```python
from build123d import *

# Parameters (mm, degrees)
SKIZZE1_W                            = 100
SKIZZE1_H                            = 50
SKIZZE1_W_2                          = 20
SKIZZE1_H_2                          = 3
AUFSATZ_LINEAR_AUSTRAGEN1_DEPTH      = 3
SKIZZE2_W                            = 90
SKIZZE2_H                            = 25
AUFSATZ_LINEAR_AUSTRAGEN2_DEPTH      = 5
SCHNITT_LINEAR_AUSTRAGEN1_DEPTH      = 4
SKIZZE4_W                            = 6
SKIZZE4_H                            = 16
SCHNITT_LINEAR_AUSTRAGEN2_DEPTH      = 5
SCHNITT_LINEAR_AUSTRAGEN2_DEPTH_BACK = 5
SKIZZE5_W                            = 25
SKIZZE5_H                            = 12.5
SCHNITT_LINEAR_AUSTRAGEN3_DEPTH      = 5.6
SKIZZE6_W                            = 4
SKIZZE6_H                            = 12.5
SCHNITT_LINEAR_AUSTRAGEN4_DEPTH      = 6.6
SCHNITT_LINEAR_AUSTRAGEN4_DEPTH_BACK = 3.4
SKIZZE8_W                            = 13
SKIZZE8_H                            = 20.5
SCHNITT_LINEAR_AUSTRAGEN5_DEPTH      = 5
SKIZZE9_W                            = 10
SKIZZE9_H                            = 20.5
SCHNITT_LINEAR_AUSTRAGEN6_DEPTH      = 8
AUFSATZ_LINEAR_AUSTRAGEN3_DEPTH      = 1
AUFSATZ_LINEAR_AUSTRAGEN4_DEPTH      = 17
SKIZZE14_W                           = 3
SKIZZE14_H                           = 42
AUFSATZ_LINEAR_AUSTRAGEN5_DEPTH      = 3
SKIZZE15_W                           = 3
SKIZZE15_H                           = 16
SCHNITT_LINEAR_AUSTRAGEN7_DEPTH      = 3
SKIZZE16_W                           = 2
SKIZZE16_H                           = 2
AUFSATZ_LINEAR_AUSTRAGEN6_DEPTH      = 17
SKIZZE17_W                           = 2
SKIZZE17_H                           = 40
SCHNITT_LINEAR_AUSTRAGEN8_DEPTH      = 20
SKIZZE18_W                           = 35
SKIZZE18_H                           = 2
SCHNITT_LINEAR_AUSTRAGEN9_DEPTH      = 17
SKIZZE19_W                           = 2
SKIZZE19_H                           = 6
SKIZZE19_W_2                         = 4
SKIZZE19_H_2                         = 4
AUFSATZ_LINEAR_AUSTRAGEN7_DEPTH      = 17
SKIZZE20_W                           = 1
SKIZZE20_H                           = 42
AUFSATZ_LINEAR_AUSTRAGEN8_DEPTH      = 3
SKIZZE21_W                           = 2
SKIZZE21_H                           = 3
AUFSATZ_LINEAR_AUSTRAGEN9_DEPTH      = 17
SKIZZE22_W                           = 20
SKIZZE22_H                           = 3
SKIZZE22_W_2                         = 90
SKIZZE22_H_2                         = 25
AUFSATZ_LINEAR_AUSTRAGEN10_DEPTH     = 5
SKIZZE24_W                           = 2
SKIZZE24_H                           = 4
AUFSATZ_LINEAR_AUSTRAGEN11_DEPTH     = 17


with BuildPart() as part:
    # Skizze1 → Aufsatz-Linear austragen1 (new body)
    with BuildSketch(Plane.XY):
        Rectangle(SKIZZE1_W, SKIZZE1_H)
        with Locations((0, -20.5)):
            Rectangle(SKIZZE1_W_2, SKIZZE1_H_2, mode=Mode.SUBTRACT)
        with Locations((0, 20.5)):
            Rectangle(SKIZZE1_W_2, SKIZZE1_H_2, mode=Mode.SUBTRACT)
    extrude(amount=AUFSATZ_LINEAR_AUSTRAGEN1_DEPTH)

    # Skizze2 → Aufsatz-Linear austragen2 (add)
    with BuildSketch(Plane(origin=(0, 0, 0), x_dir=(-1, 0, 0), z_dir=(0, 0, -1))):
        Rectangle(SKIZZE2_W, SKIZZE2_H)
    extrude(amount=AUFSATZ_LINEAR_AUSTRAGEN2_DEPTH)

    # Skizze3 → Schnitt-Linear austragen1 (cut)
    with BuildSketch(Plane(origin=(0, 0, -5), x_dir=(-1, 0, 0), z_dir=(0, 0, -1))):
        with BuildLine():
            Line((33, -8), (13, -8))
            Line((13, -8), (13, 8))
            Line((13, 8), (33, 8))
            ThreePointArc((33, 8), (41, 0), (33, -8))
        make_face()
    extrude(amount=-SCHNITT_LINEAR_AUSTRAGEN1_DEPTH, mode=Mode.SUBTRACT)

    # Skizze4 → Schnitt-Linear austragen2 (cut, two sides)
    with BuildSketch(Plane(origin=(0, 0, -1), x_dir=(-1, 0, 0), z_dir=(0, 0, -1))) as schnitt_linear_austragen2_sk:
        with Locations((16, 0)):
            Rectangle(SKIZZE4_W, SKIZZE4_H)
    extrude(amount=SCHNITT_LINEAR_AUSTRAGEN2_DEPTH, mode=Mode.SUBTRACT)
    extrude(schnitt_linear_austragen2_sk.sketch, amount=-SCHNITT_LINEAR_AUSTRAGEN2_DEPTH_BACK, mode=Mode.SUBTRACT)

    # Skizze5 → Schnitt-Linear austragen3 (cut)
    with BuildSketch(Plane(origin=(0, 0, -5), x_dir=(-1, 0, 0), z_dir=(0, 0, -1))):
        with Locations((-2.5, 0)):
            Rectangle(SKIZZE5_W, SKIZZE5_H)
    extrude(amount=-SCHNITT_LINEAR_AUSTRAGEN3_DEPTH, mode=Mode.SUBTRACT)

    # Skizze6 → Schnitt-Linear austragen4 (cut, two sides)
    with BuildSketch(Plane(origin=(0, 0, 0.6), x_dir=(-1, 0, 0), z_dir=(0, 0, -1))) as schnitt_linear_austragen4_sk:
        with Locations((8, 0)):
            Rectangle(SKIZZE6_W, SKIZZE6_H)
    extrude(amount=SCHNITT_LINEAR_AUSTRAGEN4_DEPTH, mode=Mode.SUBTRACT)
    extrude(schnitt_linear_austragen4_sk.sketch, amount=-SCHNITT_LINEAR_AUSTRAGEN4_DEPTH_BACK, mode=Mode.SUBTRACT)

    # Skizze8 → Schnitt-Linear austragen5 (cut)
    with BuildSketch(Plane.XY.offset(3)):
        with Locations((35.5, 0)):
            Rectangle(SKIZZE8_W, SKIZZE8_H)
    extrude(amount=-SCHNITT_LINEAR_AUSTRAGEN5_DEPTH, mode=Mode.SUBTRACT)

    # Skizze9 → Schnitt-Linear austragen6 (cut)
    with BuildSketch(Plane.XY.offset(3)):
        with Locations((24, 0)):
            Rectangle(SKIZZE9_W, SKIZZE9_H)
    extrude(amount=-SCHNITT_LINEAR_AUSTRAGEN6_DEPTH, mode=Mode.SUBTRACT)

    # Skizze10 → Aufsatz-Linear austragen3 (add)
    with BuildSketch(Plane(origin=(0, 0, -5), x_dir=(-1, 0, 0), z_dir=(0, 0, -1))):
        with BuildLine():
            Line((38.291502622, -6), (38.291502622, 6))
            ThreePointArc((38.291502622, 6), (41, 0), (38.291502622, -6))
        make_face()
    extrude(amount=-AUFSATZ_LINEAR_AUSTRAGEN3_DEPTH)

    # Skizze11 → Aufsatz-Linear austragen4 (add)
    with BuildSketch(Plane.XY.offset(3)):
        Polygon((-50, 25), (-50, -25), (-48, -25), (-11, -25), (-11, -23), (-48, -23), (-48, 25), align=None)
        Polygon((50, -25), (50, 25), (48, 25), (48, -23), (11, -23), (11, -25), align=None)
    extrude(amount=AUFSATZ_LINEAR_AUSTRAGEN4_DEPTH)

    # Skizze14 → Aufsatz-Linear austragen5 (add)
    with BuildSketch(Plane.XY.offset(3)):
        with Locations((-11.5, 0)):
            Rectangle(SKIZZE14_W, SKIZZE14_H)
        with Locations((45.5, 0)):
            Rectangle(SKIZZE14_W, SKIZZE14_H)
    extrude(amount=AUFSATZ_LINEAR_AUSTRAGEN5_DEPTH)

    # Skizze15 → Schnitt-Linear austragen7 (cut)
    with BuildSketch(Plane.XY.offset(6)):
        with Locations((-11.5, 0)):
            Rectangle(SKIZZE15_W, SKIZZE15_H)
    extrude(amount=-SCHNITT_LINEAR_AUSTRAGEN7_DEPTH, mode=Mode.SUBTRACT)

    # Skizze16 → Aufsatz-Linear austragen6 (add)
    with BuildSketch(Plane.XY.offset(3)):
        with Locations((-47, -22)):
            Rectangle(SKIZZE16_W, SKIZZE16_H)
        with Locations((47, -22)):
            Rectangle(SKIZZE16_W, SKIZZE16_H)
    extrude(amount=AUFSATZ_LINEAR_AUSTRAGEN6_DEPTH)

    # Skizze17 → Schnitt-Linear austragen8 (cut)
    with BuildSketch(Plane.XY.offset(20)):
        with Locations((-49, -1)):
            Rectangle(SKIZZE17_W, SKIZZE17_H)
        with Locations((49, -1)):
            Rectangle(SKIZZE17_W, SKIZZE17_H)
    extrude(amount=-SCHNITT_LINEAR_AUSTRAGEN8_DEPTH, mode=Mode.SUBTRACT)

    # Skizze18 → Schnitt-Linear austragen9 (cut)
    with BuildSketch(Plane.XY.offset(20)):
        with Locations((28.5, -24)):
            Rectangle(SKIZZE18_W, SKIZZE18_H)
    extrude(amount=-SCHNITT_LINEAR_AUSTRAGEN9_DEPTH, mode=Mode.SUBTRACT)

    # Skizze19 → Aufsatz-Linear austragen7 (add)
    with BuildSketch(Plane.XY.offset(3)):
        with Locations((-47, 22)):
            Rectangle(SKIZZE19_W, SKIZZE19_H)
        with Locations((46, 23)):
            Rectangle(SKIZZE19_W_2, SKIZZE19_H_2)
    extrude(amount=AUFSATZ_LINEAR_AUSTRAGEN7_DEPTH)

    # Skizze20 → Aufsatz-Linear austragen8 (add)
    with BuildSketch(Plane.XY.offset(3)):
        with Locations((47.5, 0)):
            Rectangle(SKIZZE20_W, SKIZZE20_H)
    extrude(amount=AUFSATZ_LINEAR_AUSTRAGEN8_DEPTH)

    # Skizze21 → Aufsatz-Linear austragen9 (add)
    with BuildSketch(Plane.XY.offset(3)):
        with Locations((-45, 23.5)):
            Rectangle(SKIZZE21_W, SKIZZE21_H)
    extrude(amount=AUFSATZ_LINEAR_AUSTRAGEN9_DEPTH)

    # Skizze22 → Aufsatz-Linear austragen10 (add)
    with BuildSketch(Plane(origin=(0, 0, 0), x_dir=(-1, 0, 0), z_dir=(0, 0, -1))):
        Polygon((-50, 19), (-50, 25), (50, 25), (50, 19), (48, 19), (48, -21), (50, -21), (50, -25), (-50, -25), (-50, -21), (-48, -21), (-48, 19), align=None)
        with Locations((0, 20.5)):
            Rectangle(SKIZZE22_W, SKIZZE22_H, mode=Mode.SUBTRACT)
        Rectangle(SKIZZE22_W_2, SKIZZE22_H_2, mode=Mode.SUBTRACT)
        with Locations((0, -20.5)):
            Rectangle(SKIZZE22_W, SKIZZE22_H, mode=Mode.SUBTRACT)
    extrude(amount=AUFSATZ_LINEAR_AUSTRAGEN10_DEPTH)

    # Skizze24 → Aufsatz-Linear austragen11 (add)
    with BuildSketch(Plane.XY.offset(3)):
        with Locations((45, -23)):
            Rectangle(SKIZZE24_W, SKIZZE24_H)
    extrude(amount=AUFSATZ_LINEAR_AUSTRAGEN11_DEPTH)


solid = part.part
```
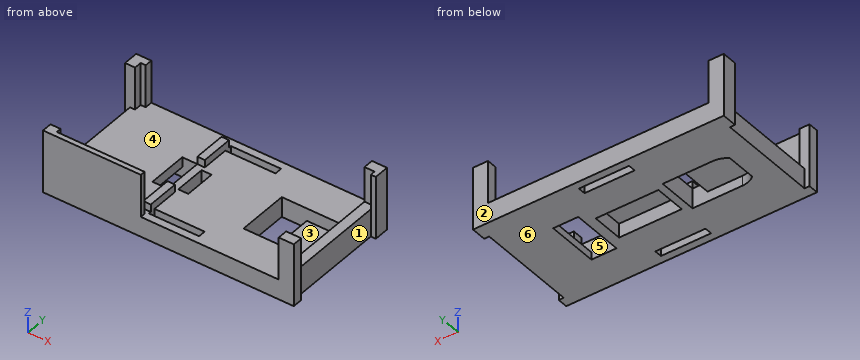
Input: part model. Units: mm. Frame: model coordinates. Face numbers are marked on the shaded views. A direction names the side the tool comes from. Coordinates: 2 decimals unless noted, no trailing zeros. Loops run counter-clockwise (first coordinate to the right, second up) from the corner with the lowest first, then second, coordinate; pieces in that order, holes last. Notation, with made-up numbers: M 6.5,-12 L 36.5,-12 A19 cw 36.5,4 Z; hole C 84,9 d4. An arc over 180 degrees is marked long. One line per item, written item: value.
(1) Section A-A (y = 0). Output: boundary loops of the cut face in (x, z), and give its area (3 significant figures).
Filled in:
outline: M -48,-5 L -38.29,-5 L -38.29,-4 L -41,-4 L -41,-1 L -19,-1 L -19,3 L -48,3 Z; M -13,-5 L -10,-5 L -10,3 L -13,3 Z; M -6,0.6 L 15,0.6 L 15,-5 L 19,-5 L 19,3 L -6,3 Z; M 29,-5 L 48,-5 L 48,6 L 44,6 L 44,3 L 42,3 L 42,-2 L 29,-2 Z
area: 352 mm^2
(2) Section D-D (x = -39.5). Output: boundary loops of the cut face in (y, z).
Filled in:
outline: M -25,-5 L 25,-5 L 25,3 L -23,3 L -23,20 L -25,20 Z; hole M -4.66,-4 L 4.66,-4 L 4.66,-1 L -4.66,-1 Z
(3) Pull-direction query (X, two-part tool) for the marked faces 1, 2, 3 and 4; classes: +X half, -X half, draft (parallel to the pull), parting line (faces both ways), or undercut.
Filled in:
face 1: +X half
face 2: draft
face 3: undercut
face 4: undercut
(4) Section C-C (z = 17). Output: boundary loops of the cut face in (x, y), and give its area (3 significant figures).
Filled in:
outline: M -50,-25 L -11,-25 L -11,-23 L -46,-23 L -46,-21 L -50,-21 Z; M -50,19 L -46,19 L -46,22 L -44,22 L -44,25 L -50,25 Z; M 44,-25 L 50,-25 L 50,-21 L 44,-21 Z; M 44,21 L 48,21 L 48,19 L 50,19 L 50,25 L 44,25 Z
area: 168 mm^2
(5) Pin query (flat end, axial travel): pin 1 (4 mm diameter, centred on x = 6, y = 0.5, fed in from -Z); pin 2 (3 mm diameter, centred on x = 8.5, y = 20, fed in from +Z); pin 3 (2.5 mm diameter, centred on x = -11.5, y = 14.5, fed in from +Z). Return the tip coordinate at first contact, or that it passes through.
Filled in:
pin 1: z = 0.6
pin 2: z = 3
pin 3: z = 6
(6) Line query: line 1 along X through (y, z) = (2, 0); line 2 along Y through (x, z) = (7, -3); line 3 along Y through (x, z) = (11, -2.75). Output: solid intervals per line, ascending. Write a range as from..to.
Filled in:
line 1: -48..-19, -13..-10, 15..19, 42..48
line 2: -25..-22, -19..-6.25, 6.25..19, 22..25
line 3: -25..-6.25, 6.25..25
(7) Section B-B (x = 9). Output: boundary loops of the cut face in (y, z), and give its area (3 significant figures).
Filled in:
outline: M -25,-5 L -22,-5 L -22,3 L -25,3 Z; M -19,-5 L -6.25,-5 L -6.25,0.6 L 6.25,0.6 L 6.25,-5 L 19,-5 L 19,3 L -19,3 Z; M 22,-5 L 25,-5 L 25,3 L 22,3 Z
area: 282 mm^2
(8) Reachability of the marked faces 5 and 6 from +Z, -Z, +X, -X, +Y, -Y: full face, straight path, thin tool, end or side. Return the list, or none.
Filled in:
face 5: +Z
face 6: -Z, +X, -X, +Y, -Y
